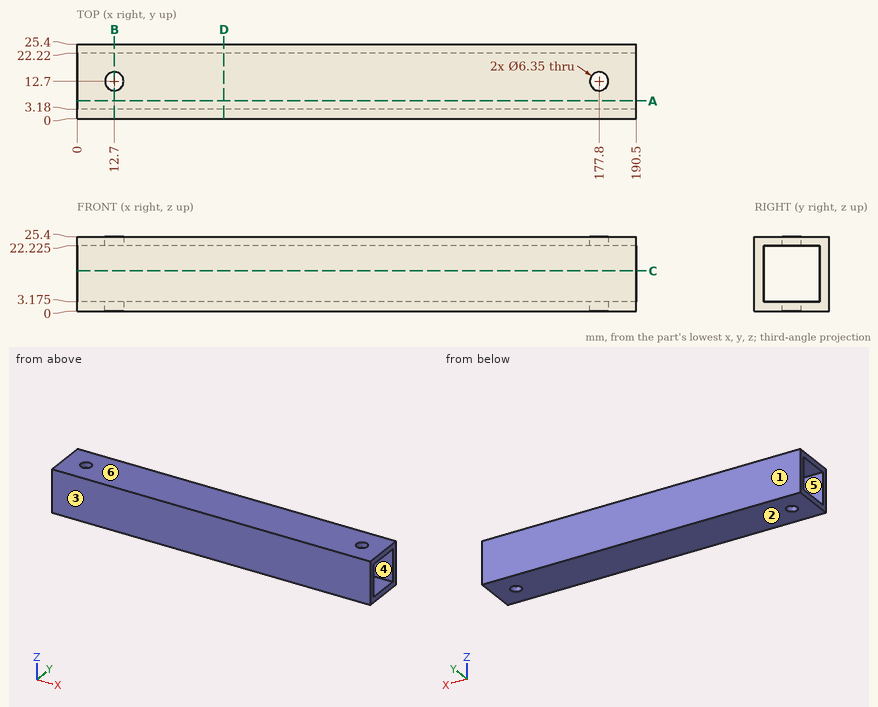
Geometry: see drawing. Coordinates: mm, zero at the bounding-box minimum. A direction names the side the tool comes from. Give positions to 0.01 mm unless a question says otherwise; leave off trailing zeros. Loops run counter-clockwise (first coordinate to the right, second up) from the corner with the lowest first, then second, coordinate; pieces in that order, holes last. Notation, with made-up numbers: (29.5, -17.5) -> (49.5, -17.5) arc R7 cw to (49.5, -10.5) -> close; hole circle Ø2 at (-21, -35). An arc over 180 degrees is marked (long way). Put each result on its own line as item: value.
1. Pull-direction query (Y, two-part tool) for the marked faces 1, 2, 3 and 4; classes: released by +Y, released by -Y, zero draft, split by the parting line, or undercut.
Taken from the geometry:
face 1: released by +Y
face 2: zero draft
face 3: released by -Y
face 4: undercut
2. Set-up query: the marked faces 5 and 6. Return all of +Z, -Z, +X, -X, +Y, -Y with unobstructed straight access to the full face (end or side cutting, diameter ignored); none if empty.
Taken from the geometry:
face 5: +X, -X
face 6: +Z, +X, -X, +Y, -Y
3. Cut plane D-D (x = 50). Return the cut outline in (y, z) (1 decimal).
Taken from the geometry:
outline: (0, 0) -> (25.4, 0) -> (25.4, 25.4) -> (0, 25.4) -> close; hole (3.2, 3.2) -> (22.2, 3.2) -> (22.2, 22.2) -> (3.2, 22.2) -> close
4. Ray query, line 1 along Z through (x, y) = (77, 17.75) (1 decimal); line 2 along Y through (x, z) = (89, 5.25); line 3 along Y through (x, z) = (177.8, 1.95) (1 decimal). Return the intervals inside material, ascending. Write a range as [from, to].
Taken from the geometry:
line 1: z = [0, 3.2], [22.2, 25.4]
line 2: y = [0, 3.18], [22.22, 25.4]
line 3: y = [0, 9.5], [15.9, 25.4]
5. Pin query (flat end, axial travel): P1, Ø5, axis at x = 12.7, y = 12.7, coming from the -Z side. Return the tip coordinate at first contact, or that it passes through.
Taken from the geometry:
P1: passes through
6. Cut plane B-B (x = 12.7). Return the cut outline in (y, z) (1 decimal), plus the area to 3 significant figures.
Taken from the geometry:
outline: (0, 0) -> (9.5, 0) -> (9.5, 3.2) -> (3.2, 3.2) -> (3.2, 22.2) -> (9.5, 22.2) -> (9.5, 25.4) -> (0, 25.4) -> close; (15.9, 0) -> (25.4, 0) -> (25.4, 25.4) -> (15.9, 25.4) -> (15.9, 22.2) -> (22.2, 22.2) -> (22.2, 3.2) -> (15.9, 3.2) -> close
area: 242 mm2
7. Cut plane C-C (z = 13.75). Return the cut outline in (x, y).
Taken from the geometry:
outline: (0, 0) -> (190.5, 0) -> (190.5, 3.18) -> (0, 3.18) -> close; (0, 22.22) -> (190.5, 22.22) -> (190.5, 25.4) -> (0, 25.4) -> close
8. Cut plane A-A (y = 6). Return the cut outline in (x, z) (1 decimal).
Taken from the geometry:
outline: (0, 0) -> (190.5, 0) -> (190.5, 3.2) -> (0, 3.2) -> close; (0, 22.2) -> (190.5, 22.2) -> (190.5, 25.4) -> (0, 25.4) -> close
